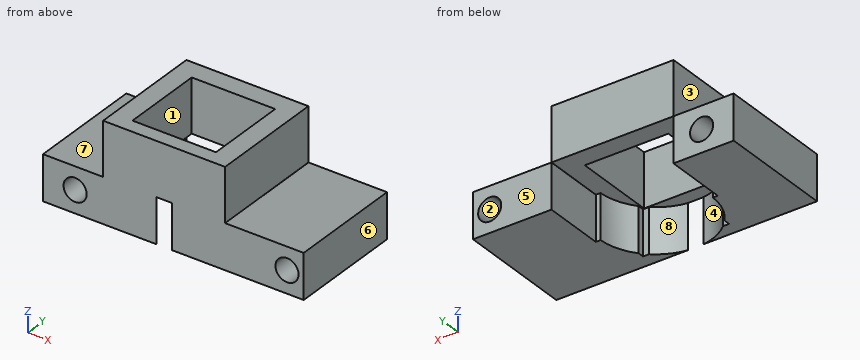
```python
from build123d import *

# Parameters (mm, degrees)
BOSS_EXTRUDE1_DEPTH   = 7
BOSS_EXTRUDE1_2_DEPTH = 7
SKETCH2_W             = 19.000397442
SKETCH2_H             = 18
SKETCH2_W_2           = 13
SKETCH2_H_2           = 12.8
BOSS_EXTRUDE2_DEPTH   = 8.35
SKETCH3_R             = 1.8
CUT_EXTRUDE1_DEPTH    = 47.557840371


with BuildPart() as part:
    # Sketch1 → Boss-Extrude1 (new body)
    with BuildSketch(Plane.XY):
        with BuildLine():
            Line((-0.5, 19.7), (-0.5, 1.7))
            Line((-0.5, 1.7), (17.158948763, 1.7))
            ThreePointArc((17.158948763, 1.7), (14.736483801, 2.411824757), (12.618126572, 3.785721996))
            Line((12.618126572, 3.785721996), (11.684321255, 3.785721996))
            Line((11.684321255, 3.785721996), (11.684321255, 4.740579311))
            ThreePointArc((11.684321255, 4.740579311), (10.208452966, 7.257442509), (9.642129796, 10.119620985))
            Line((9.642129796, 10.119620985), (8.884321255, 10.119620985))
            Line((8.884321255, 10.119620985), (8.884321255, 19.7))
            Line((8.884321255, 19.7), (-0.5, 19.7))
        make_face()
    extrude(amount=BOSS_EXTRUDE1_DEPTH)



with BuildPart() as body_2:
    # Sketch1 → Boss-Extrude1 2 (new body)
    with BuildSketch(Plane.XY):
        with BuildLine():
            ThreePointArc((24.159354013, 3.785721996), (22.040996783, 2.411824757), (19.618531821, 1.7))
            Line((19.618531821, 1.7), (40.1, 1.7))
            Line((40.1, 1.7), (40.1, 19.7))
            Line((40.1, 19.7), (27.884321255, 19.7))
            Line((27.884321255, 19.7), (27.884321255, 10.119620985))
            Line((27.884321255, 10.119620985), (27.135350788, 10.119620985))
            ThreePointArc((27.135350788, 10.119620985), (26.566586462, 7.25102021), (25.084321255, 4.730057473))
            Line((25.084321255, 4.730057473), (25.084321255, 3.785721996))
            Line((25.084321255, 3.785721996), (24.159354013, 3.785721996))
        make_face()
    extrude(amount=BOSS_EXTRUDE1_2_DEPTH)


with BuildPart() as part_1:
    add(part.part)

    add(body_2.part)  # Boss-Extrude2 merges body 2
    # Sketch2 → Boss-Extrude2 (add)
    with BuildSketch(Plane.XY.offset(7)):
        with Locations((18.360198721, 10.7)):
            Rectangle(SKETCH2_W, SKETCH2_H)
        with Locations((18.360397442, 10.287463183)):
            Rectangle(SKETCH2_W_2, SKETCH2_H_2, mode=Mode.SUBTRACT)
    extrude(amount=BOSS_EXTRUDE2_DEPTH)

    # Sketch3 → Cut-Extrude1 (cut, through all)
    with BuildSketch(Plane(origin=(0, 19.7, 0), x_dir=(1, 0, 0), z_dir=(0, 1, 0))):
        with Locations(Location((4.5, -3.5, 0), (0, 0, 270))):
            Circle(SKETCH3_R)
        with Locations(Location((37.5, -3.5, 0), (0, 0, 270))):
            Circle(SKETCH3_R)
    extrude(amount=-CUT_EXTRUDE1_DEPTH, mode=Mode.SUBTRACT)


solid = part_1.part
```
Geometry: final body of the model. Coordinates: model frame, mm. Face numbers are marked on the shaded views. A direction names the side the tool comes from. Coordinates: 2 decimals unless noted, no trailing zeros. Order: outer loops, then holes, each group sorted by start corner. A loop starts at its lowest first (then second) coordinate and runs counter-clockwise, first axis right, second up. Notation, with made-up numbers: (11, 27) - (65, 27) arc R25 cw to (65, 41) - close; hole circle Ø3 at (38, 73). An arc over 180 degrees is marked (long way). Return JSON: item names as keys, results as strings. Group by question number.
1. Cut plane B-B (y = 12). Output: boundary loops of the cut face in (x, z).
2. Material intervals for line 1 along X through (y, z) = (12.5, 3.5); line 2 along X through (y, z) = (15.5, 4); line 3 along Y through (x, z) = (17.5, 7.5), sorted ascending. Write a range as [from, to].
3. Pin query (flat end, axial travel): pin 1 (0.7 mm diameter, centred on x = 24.5, z = 3, fed in from +Y); pin 2 (0.6 mm diameter, centred on x = 9.5, z = 3, fed in from +Y); pin 3 (3 mm diameter, centred on x = 3.5, y = 8, fed in from +Z); pin 4 (3 mm diameter, centred on x = 4.5, z = 3.5, fed in from +Y). Return the tip coordinate at first contact, or that it passes through.
4. Set-up query: the marked faces 1, 2, 3, 4 and 5. Return all of +Z, -Z, +X, -X, +Y, -Y with unobstructed straight access to the full face (end or side cutting, diameter ignored); none if empty.
5. Cut plane C-C (z = 3.5). Output: boundary loops of the cut face in (x, y).
6. Pull-direction query (X, two-part tool) for the marked faces 6, 7 and 8; classes: pulls with the +X half, pulls with the -X half, needs draft (parallel to the pull), parting line crosses it, or undercut.
7. Cut plane A-A (y = 18.5). Output: boundary loops of the cut face in (x, z), plus the area to 3 significant figures.
8. Cut plane D-D (x = 4.5). Output: boundary loops of the cut face in (y, z).
Resolved:
{
 "1": {"outline": "(-0.5, 0) - (8.88, 0) - (8.88, 7) - (11.86, 7) - (11.86, 15.35) - (8.86, 15.35) - (8.86, 7) - (-0.5, 7) - close; (24.86, 7) - (27.86, 7) - (27.86, 15.35) - (24.86, 15.35) - close; (27.88, 0) - (40.1, 0) - (40.1, 7) - (27.88, 7) - close; hole circle Ø3.6 at (4.5, 3.5); hole circle Ø3.6 at (37.5, 3.5)"},
 "2": {"line 1": "x = [-0.5, 2.7], [6.3, 8.88], [27.88, 35.7], [39.3, 40.1]", "line 2": "x = [-0.5, 2.77], [6.23, 8.88], [27.88, 35.77], [39.23, 40.1]", "line 3": "y = [1.7, 3.89], [16.69, 19.7]"},
 "3": {"pin 1": "stops at y = 3.79", "pin 2": "stops at y = 10.12", "pin 3": "stops at z = 7", "pin 4": "passes through"},
 "4": {"face 1": "+Z, -Z", "face 2": "+Y, -Y", "face 3": "+Z, -X, +Y, -Y", "face 4": "-Z, +Y", "face 5": "+Z, -Z, +X, -X, +Y"},
 "5": {"outline": "(-0.5, 1.7) - (2.7, 1.7) - (2.7, 19.7) - (-0.5, 19.7) - close; (6.3, 1.7) - (17.16, 1.7) arc R8.75 cw to (12.62, 3.79) - (11.68, 3.79) - (11.68, 4.74) arc R8.75 cw to (9.64, 10.12) - (8.88, 10.12) - (8.88, 19.7) - (6.3, 19.7) - close; (19.62, 1.7) - (35.7, 1.7) - (35.7, 19.7) - (27.88, 19.7) - (27.88, 10.12) - (27.14, 10.12) arc R8.75 cw to (25.08, 4.73) - (25.08, 3.79) - (24.16, 3.79) arc R8.75 cw to start; (39.3, 1.7) - (40.1, 1.7) - (40.1, 19.7) - (39.3, 19.7) - close"},
 "6": {"face 6": "pulls with the +X half", "face 7": "needs draft", "face 8": "undercut"},
 "7": {"outline": "(-0.5, 0) - (8.88, 0) - (8.88, 7) - (27.86, 7) - (27.86, 15.35) - (8.86, 15.35) - (8.86, 7) - (-0.5, 7) - close; (27.88, 0) - (40.1, 0) - (40.1, 7) - (27.88, 7) - close; hole circle Ø3.6 at (4.5, 3.5); hole circle Ø3.6 at (37.5, 3.5)", "area": "289 mm²"},
 "8": {"outline": "(1.7, 0) - (19.7, 0) - (19.7, 1.7) - (1.7, 1.7) - close; (1.7, 5.3) - (19.7, 5.3) - (19.7, 7) - (1.7, 7) - close"}
}
